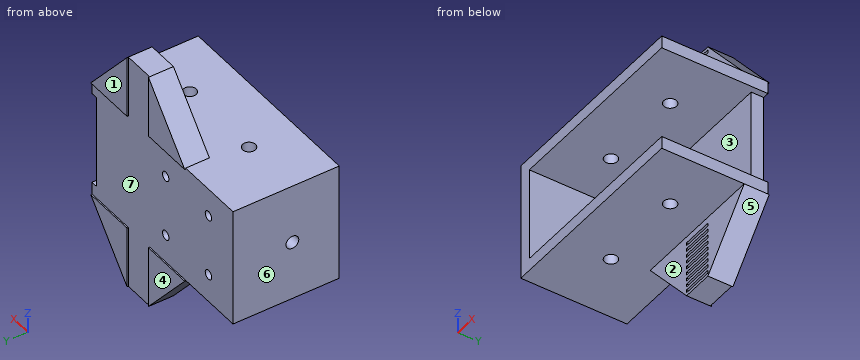
```python
from build123d import *

# Parameters (mm, degrees)
SKIZZE1_W                                  = 60
SKIZZE1_H                                  = 30.2
SKIZZE1_R                                  = 1.5
AUFSATZ_LINEAR_AUSTRAGEN1_DEPTH            = 4
LINEAR_AUSTRAGEN_D_NN1_DEPTH               = 34
F_4_1_4_1_DURCHMESSER_BOHRUNG1_D           = 4.1
F_4_1_4_1_DURCHMESSER_BOHRUNG1_ON_FACE_2_D = 4.1
SKIZZE4_W                                  = 10
SKIZZE4_H                                  = 7.6
AUFSATZ_LINEAR_AUSTRAGEN3_DEPTH            = 20
SKIZZE5_W                                  = 1
SKIZZE5_H                                  = 2
SCHNITT_LINEAR_AUSTRAGEN1_DEPTH            = 20
AUFSATZ_LINEAR_AUSTRAGEN4_DEPTH            = 8


with BuildPart() as part:
    # Skizze1 → Aufsatz-Linear austragen1 (new body)
    with BuildSketch(Plane(origin=(0, 0, 0), x_dir=(1, 0, 0), z_dir=(0, 1, 0))):
        Rectangle(SKIZZE1_W, SKIZZE1_H)
        with Locations((-22.5, 10)):
            Circle(SKIZZE1_R, mode=Mode.SUBTRACT)
        with Locations((-22.5, -10)):
            Circle(SKIZZE1_R, mode=Mode.SUBTRACT)
        with Locations((-2.5, 10)):
            Circle(SKIZZE1_R, mode=Mode.SUBTRACT)
        with Locations((-2.5, -10)):
            Circle(SKIZZE1_R, mode=Mode.SUBTRACT)
    extrude(amount=AUFSATZ_LINEAR_AUSTRAGEN1_DEPTH)

    # Skizze2 → Linear-Austragen-Dünn1 (add)
    with BuildSketch(Plane(origin=(0, 4, 0), x_dir=(1, 0, 0), z_dir=(0, 1, 0))):
        Polygon((32, -15.1), (-30, -15.1), (-30, 15.1), (32, 15.1), (32, 19.1), (-34, 19.1), (-34, -19.1), (32, -19.1), align=None)
    extrude(amount=-LINEAR_AUSTRAGEN_D_NN1_DEPTH)

    # Ø4.1 (4.1) Durchmesser Bohrung1 (through all)
    with Locations(Plane(origin=(-14, -14.808153884, -19.1), x_dir=(-1, 0, 0), z_dir=(0, 0, -1))):
        with Locations((0, 0), (-27.999342761, -0.191846116)):
            Hole(F_4_1_4_1_DURCHMESSER_BOHRUNG1_D / 2)

    # Ø4.1 (4.1) Durchmesser Bohrung1 on face 2 (through all)
    with Locations(Plane(origin=(-34, -15, 0), x_dir=(0, 0, -1), z_dir=(-1, 0, 0))):
        with Locations((0, 0)):
            Hole(F_4_1_4_1_DURCHMESSER_BOHRUNG1_ON_FACE_2_D / 2)

    # Skizze4 → Aufsatz-Linear austragen3 (add)
    with BuildSketch(Plane(origin=(0, 0, -19.1), x_dir=(-1, 0, 0), z_dir=(0, 0, -1))):
        with Locations((-10, 0.2)):
            Rectangle(SKIZZE4_W, SKIZZE4_H)
    aufsatz_linear_austragen3 = extrude(amount=AUFSATZ_LINEAR_AUSTRAGEN3_DEPTH)

    # Skizze5 → Schnitt-Linear austragen1 (cut)
    with BuildSketch(Plane(origin=(15, 0, 0), x_dir=(0, 0, -1), z_dir=(1, 0, 0))):
        with Locations((37.6, -2.6)):
            Rectangle(SKIZZE5_W, SKIZZE5_H)
        with Locations((35.6, -2.6)):
            Rectangle(SKIZZE5_W, SKIZZE5_H)
        with Locations((33.6, -2.6)):
            Rectangle(SKIZZE5_W, SKIZZE5_H)
        with Locations((31.6, -2.6)):
            Rectangle(SKIZZE5_W, SKIZZE5_H)
        with Locations((29.6, -2.6)):
            Rectangle(SKIZZE5_W, SKIZZE5_H)
        with Locations((27.6, -2.6)):
            Rectangle(SKIZZE5_W, SKIZZE5_H)
        with Locations((25.6, -2.6)):
            Rectangle(SKIZZE5_W, SKIZZE5_H)
        with Locations((23.6, -2.6)):
            Rectangle(SKIZZE5_W, SKIZZE5_H)
        with Locations((21.6, -2.6)):
            Rectangle(SKIZZE5_W, SKIZZE5_H)
    schnitt_linear_austragen1 = extrude(amount=-SCHNITT_LINEAR_AUSTRAGEN1_DEPTH, mode=Mode.SUBTRACT)

    # Skizze6 → Aufsatz-Linear austragen4 (add)
    with BuildSketch(Plane.XZ.offset(3.6)):
        Polygon((15, -39.1), (32, -19.1), (15, -19.1), align=None)
        Polygon((5, -39.1), (5, -19.1), (-12, -19.1), align=None)
    aufsatz_linear_austragen4 = extrude(amount=-AUFSATZ_LINEAR_AUSTRAGEN4_DEPTH)

    # Spiegeln1: Aufsatz-Linear austragen3, Schnitt-Linear austragen1, Aufsatz-Linear austragen4 across plane
    add(aufsatz_linear_austragen3.mirror(Plane.XY.offset(-0.1)))
    add(schnitt_linear_austragen1.mirror(Plane.XY.offset(-0.1)), mode=Mode.SUBTRACT)
    add(aufsatz_linear_austragen4.mirror(Plane.XY.offset(-0.1)))


solid = part.part
```
Could you check a few things on this model? Use its own coordinates, in mm. Face numbers are marked on the shaded views. A direction names the side the tool comes from. Round coordinates to 2 decimals unless told otherwise and drop trailing zeros. Loops run counter-clockwise (first coordinate to the right, second up) from the corner with the lowest first, then second, coordinate; pieces in that order, holes last.
Q1. I want a section at C-C (y = 2.5). Write out the boundary of the cut face in (x, z).
Q2. For P1, Ø3.5, axis at x = -22.5, z = 10, coming from the +Y side; P2, Ø3, axis at x = -10, z = 6, coming from the -Y side; P3, Ø0.5, axis at y = -2.5, z = 25.5, coming from the +X side, each with a flat end and sliding along its axis, tell me the tip position at first contact or that it passes through.
Q3. I want a section at B-B (z = 0). Write out the boundary of the cut face in (x, y).
Q4. On a 3-axis mill with a long thin cutter (end or side, diameter ignored), from which of +Z, -Z, +X, -X, +Y, -Y can I reach the whole of each face in a straight line? I mean the marked faces 1, 2 and 3. Say none if no direction works.
Q5. I want a section at A-A (x = -22.5). Write out the boundary of the cut face in (y, z).
Q6. Thinking about a two-plate mould opening in X: for the marked faces 4, 5, 6 and 7, which applies, pulls with the +X half, pulls with the -X half, needs draft (parallel to the pull), parting line crosses it, or undercut?
Q7. Please list where these lines run through material, in increasing order: L1, parallel to X at y = 1.8, z = -10; L2, parallel to Z at x = -22.5, y = 1.05; L3, parallel to Y at x = -31, z = 0.
Q8. I want a section at D-D (y = -20). Write out the boundary of the cut face in (x, z).
Answer below:
1. outline: (-34, -19.1) - (-12, -19.1) - (5, -39.1) - (15, -39.1) - (32, -19.1) - (32, -15.1) - (30, -15.1) - (30, 15.1) - (32, 15.1) - (32, 19.1) - (31.83, 19.1) - (15, 38.9) - (5, 38.9) - (-11.83, 19.1) - (-34, 19.1) - close; hole circle Ø3 at (-22.5, -10); hole circle Ø3 at (-22.5, 10); hole circle Ø3 at (-2.5, -10); hole circle Ø3 at (-2.5, 10)
2. P1: stops at y = 4
2. P2: stops at y = 0
2. P3: stops at x = 26.6
3. outline: (-34, -30) - (-30, -30) - (-30, -17.05) - (-34, -17.05) - close; (-34, -12.95) - (-30, -12.95) - (-30, 0) - (30, 0) - (30, 4) - (-34, 4) - close
4. face 1: +Z, -Z, +X, -X, +Y
4. face 2: -Z, +X, -X, -Y
4. face 3: +X, -Y
5. outline: (-30, -19.1) - (4, -19.1) - (4, -11.5) - (0, -11.5) - (0, -15.1) - (-30, -15.1) - close; (-30, 15.1) - (0, 15.1) - (0, 11.5) - (4, 11.5) - (4, 19.1) - (-30, 19.1) - close; (0, -8.5) - (4, -8.5) - (4, 8.5) - (0, 8.5) - close
6. face 4: needs draft
6. face 5: pulls with the +X half
6. face 6: pulls with the -X half
6. face 7: undercut
7. L1: x = -34 to -24, -21 to -4, -1 to 30
7. L2: z = -19.1 to -11.5, -8.5 to 8.5, 11.5 to 19.1
7. L3: y = -30 to -17.05, -12.95 to 4
8. outline: (-34, -19.1) - (32, -19.1) - (32, -15.1) - (-30, -15.1) - (-30, 15.1) - (32, 15.1) - (32, 19.1) - (-34, 19.1) - close
